Check sheet for the modelled part. Datum: model origin and axes. Units: mm. Face numbers are marked on the shaded views. A direction names the side the tool comes from. Give positions to 0.01 mm unless a question says otherwise; leave off trailing zeros. Loops run counter-clockwise (first coordinate to the right, second up) from the corner with the lowest first, then second, coordinate; pieces in that order, holes last. Notation, with made-up numbers: M -15,-25 L 13,-25 A20 ccw 13,-16 Z; hole C 31,18 d8. An arc over 180 degrees is marked long. Use one line per item in the form item = value.
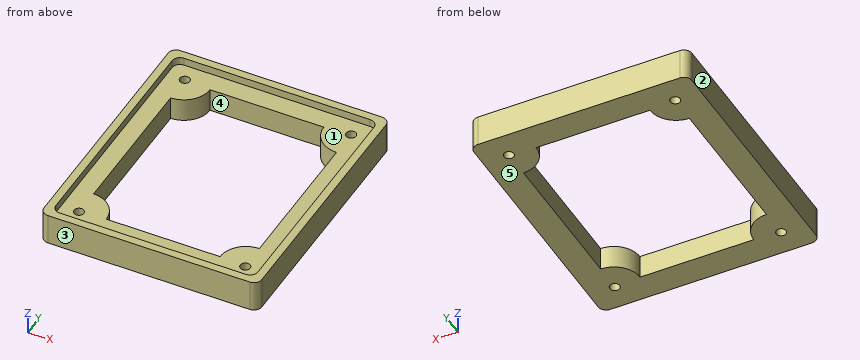
from build123d import *

# Parameters (mm, degrees)
F1_DEPTH = 6
F2_DEPTH = 8
F4_D     = 2.5
F4_DEPTH = 150
F4_TIP   = 0.7510757738
F5_R     = 2


with BuildPart() as f1:
    # F0 (on Top) → F1 (new body)
    with BuildSketch(Plane.XY):
        with BuildLine():
            Line((-20.9328360941, 18.9328360941), (-20.9328360941, 25.5))
            Line((-20.9328360941, 25.5), (-14.3656721882, 25.5))
            ThreePointArc((-14.3656721882, 25.5), (-14.9709415927, 28.2538074954), (-16.6751792541, 30.5))
            Line((-16.6751792541, 30.5), (-25.1904929341, 30.5))
            ThreePointArc((-25.1904929341, 30.5), (-25.3474833162, 30.3619473127), (-25.5, 30.2189676438))
            Line((-25.5, 30.2189676438), (-25.5, 20.7810323562))
            ThreePointArc((-25.5, 20.7810323562), (-23.3963100419, 19.4123947339), (-20.9328360941, 18.9328360941))
        make_face()
        with BuildLine():
            Line((-14.3656721882, 25.5), (-20.9328360941, 25.5))
            Line((-20.9328360941, 25.5), (-20.9328360941, 18.9328360941))
            ThreePointArc((-20.9328360941, 18.9328360941), (-16.289149963, 20.856313869), (-14.3656721882, 25.5))
        make_face()
        with BuildLine():
            ThreePointArc((-16.6751792541, 30.5), (-14.9709415927, 28.2538074954), (-14.3656721882, 25.5))
            Line((-14.3656721882, 25.5), (14.3656721882, 25.5))
            ThreePointArc((14.3656721882, 25.5), (14.9709415927, 28.2538074954), (16.6751792541, 30.5))
            Line((16.6751792541, 30.5), (-16.6751792541, 30.5))
        make_face()
        with BuildLine():
            ThreePointArc((16.6751792541, 30.5), (14.9709415927, 28.2538074954), (14.3656721882, 25.5))
            Line((14.3656721882, 25.5), (20.9328360941, 25.5))
            Line((20.9328360941, 25.5), (20.9328360941, 18.9328360941))
            ThreePointArc((20.9328360941, 18.9328360941), (23.3963100419, 19.4123947339), (25.5, 20.7810323562))
            Line((25.5, 20.7810323562), (25.5, 30.2189676438))
            ThreePointArc((25.5, 30.2189676438), (25.3474833162, 30.3619473127), (25.1904929341, 30.5))
            Line((25.1904929341, 30.5), (16.6751792541, 30.5))
        make_face()
        with BuildLine():
            Line((20.9328360941, 25.5), (14.3656721882, 25.5))
            ThreePointArc((14.3656721882, 25.5), (16.289149963, 20.856313869), (20.9328360941, 18.9328360941))
            Line((20.9328360941, 18.9328360941), (20.9328360941, 25.5))
        make_face()
        with BuildLine():
            ThreePointArc((25.5, 20.7810323562), (23.3963100419, 19.4123947339), (20.9328360941, 18.9328360941))
            Line((20.9328360941, 18.9328360941), (20.9328360941, -18.9328360941))
            ThreePointArc((20.9328360941, -18.9328360941), (23.3963100419, -19.4123947339), (25.5, -20.7810323562))
            Line((25.5, -20.7810323562), (25.5, 20.7810323562))
        make_face()
        with BuildLine():
            ThreePointArc((25.5, -20.7810323562), (23.3963100419, -19.4123947339), (20.9328360941, -18.9328360941))
            Line((20.9328360941, -18.9328360941), (20.9328360941, -25.5))
            Line((20.9328360941, -25.5), (14.3656721882, -25.5))
            ThreePointArc((14.3656721882, -25.5), (14.9709415927, -28.2538074954), (16.6751792541, -30.5))
            Line((16.6751792541, -30.5), (25.1904929341, -30.5))
            ThreePointArc((25.1904929341, -30.5), (25.3474833162, -30.3619473127), (25.5, -30.2189676438))
            Line((25.5, -30.2189676438), (25.5, -20.7810323562))
        make_face()
        with BuildLine():
            Line((20.9328360941, -25.5), (20.9328360941, -18.9328360941))
            ThreePointArc((20.9328360941, -18.9328360941), (16.289149963, -20.856313869), (14.3656721882, -25.5))
            Line((14.3656721882, -25.5), (20.9328360941, -25.5))
        make_face()
        with BuildLine():
            Line((-20.9328360941, -25.5), (-20.9328360941, -18.9328360941))
            ThreePointArc((-20.9328360941, -18.9328360941), (-23.3963100419, -19.4123947339), (-25.5, -20.7810323562))
            Line((-25.5, -20.7810323562), (-25.5, -30.2189676438))
            ThreePointArc((-25.5, -30.2189676438), (-25.3474833162, -30.3619473127), (-25.1904929341, -30.5))
            Line((-25.1904929341, -30.5), (-16.6751792541, -30.5))
            ThreePointArc((-16.6751792541, -30.5), (-14.9709415927, -28.2538074954), (-14.3656721882, -25.5))
            Line((-14.3656721882, -25.5), (-20.9328360941, -25.5))
        make_face()
        with BuildLine():
            ThreePointArc((-14.3656721882, -25.5), (-16.289149963, -20.856313869), (-20.9328360941, -18.9328360941))
            Line((-20.9328360941, -18.9328360941), (-20.9328360941, -25.5))
            Line((-20.9328360941, -25.5), (-14.3656721882, -25.5))
        make_face()
        with BuildLine():
            Line((-20.9328360941, -18.9328360941), (-20.9328360941, 18.9328360941))
            ThreePointArc((-20.9328360941, 18.9328360941), (-23.3963100419, 19.4123947339), (-25.5, 20.7810323562))
            Line((-25.5, 20.7810323562), (-25.5, -20.7810323562))
            ThreePointArc((-25.5, -20.7810323562), (-23.3963100419, -19.4123947339), (-20.9328360941, -18.9328360941))
        make_face()
        with BuildLine():
            Line((14.3656721882, -25.5), (-14.3656721882, -25.5))
            ThreePointArc((-14.3656721882, -25.5), (-14.9709415927, -28.2538074954), (-16.6751792541, -30.5))
            Line((-16.6751792541, -30.5), (16.6751792541, -30.5))
            ThreePointArc((16.6751792541, -30.5), (14.9709415927, -28.2538074954), (14.3656721882, -25.5))
        make_face()
        with BuildLine():
            Line((25.5, 30.5), (25.1904929341, 30.5))
            ThreePointArc((25.1904929341, 30.5), (25.3474833162, 30.3619473127), (25.5, 30.2189676438))
            Line((25.5, 30.2189676438), (25.5, 30.5))
        make_face()
        with BuildLine():
            ThreePointArc((-25.5, 30.2189676438), (-25.3474833162, 30.3619473127), (-25.1904929341, 30.5))
            Line((-25.1904929341, 30.5), (-25.5, 30.5))
            Line((-25.5, 30.5), (-25.5, 30.2189676438))
        make_face()
        with BuildLine():
            ThreePointArc((-25.1904929341, -30.5), (-25.3474833162, -30.3619473127), (-25.5, -30.2189676438))
            Line((-25.5, -30.2189676438), (-25.5, -30.5))
            Line((-25.5, -30.5), (-25.1904929341, -30.5))
        make_face()
        with BuildLine():
            Line((25.5, -30.5), (25.5, -30.2189676438))
            ThreePointArc((25.5, -30.2189676438), (25.3474833162, -30.3619473127), (25.1904929341, -30.5))
            Line((25.1904929341, -30.5), (25.5, -30.5))
        make_face()
    extrude(amount=F1_DEPTH)

    # F0 (on Top) → F2 (join)
    with BuildSketch(Plane.XY):
        with BuildLine():
            ThreePointArc((-25.1904929341, 30.5), (-20.9328360941, 32.0671639059), (-16.6751792541, 30.5))
            Line((-16.6751792541, 30.5), (16.6751792541, 30.5))
            ThreePointArc((16.6751792541, 30.5), (20.9328360941, 32.0671639059), (25.1904929341, 30.5))
            Line((25.1904929341, 30.5), (25.5, 30.5))
            Line((25.5, 30.5), (25.5, 30.2189676438))
            ThreePointArc((25.5, 30.2189676438), (26.9793621927, 28.062647831), (27.5, 25.5))
            Line((27.5, 25.5), (27.5, 32.5))
            Line((27.5, 32.5), (-27.5, 32.5))
            Line((-27.5, 32.5), (-27.5, 25.5))
            ThreePointArc((-27.5, 25.5), (-26.9793621927, 28.062647831), (-25.5, 30.2189676438))
            Line((-25.5, 30.2189676438), (-25.5, 30.5))
            Line((-25.5, 30.5), (-25.1904929341, 30.5))
        make_face()
        with BuildLine():
            Line((-25.1904929341, 30.5), (-16.6751792541, 30.5))
            ThreePointArc((-16.6751792541, 30.5), (-20.9328360941, 32.0671639059), (-25.1904929341, 30.5))
        make_face()
        with BuildLine():
            ThreePointArc((-27.5, 25.5), (-26.9793621927, 22.937352169), (-25.5, 20.7810323562))
            Line((-25.5, 20.7810323562), (-25.5, 30.2189676438))
            ThreePointArc((-25.5, 30.2189676438), (-26.9793621927, 28.062647831), (-27.5, 25.5))
        make_face()
        with BuildLine():
            Line((-25.5, -20.7810323562), (-25.5, 20.7810323562))
            ThreePointArc((-25.5, 20.7810323562), (-26.9793621927, 22.937352169), (-27.5, 25.5))
            Line((-27.5, 25.5), (-27.5, -25.5))
            ThreePointArc((-27.5, -25.5), (-26.9793621927, -22.937352169), (-25.5, -20.7810323562))
        make_face()
        with BuildLine():
            Line((-25.5, -30.2189676438), (-25.5, -20.7810323562))
            ThreePointArc((-25.5, -20.7810323562), (-26.9793621927, -22.937352169), (-27.5, -25.5))
            ThreePointArc((-27.5, -25.5), (-26.9793621927, -28.062647831), (-25.5, -30.2189676438))
        make_face()
        with BuildLine():
            Line((16.6751792541, -30.5), (-16.6751792541, -30.5))
            ThreePointArc((-16.6751792541, -30.5), (-20.9328360941, -32.0671639059), (-25.1904929341, -30.5))
            Line((-25.1904929341, -30.5), (-25.5, -30.5))
            Line((-25.5, -30.5), (-25.5, -30.2189676438))
            ThreePointArc((-25.5, -30.2189676438), (-26.9793621927, -28.062647831), (-27.5, -25.5))
            Line((-27.5, -25.5), (-27.5, -32.5))
            Line((-27.5, -32.5), (27.5, -32.5))
            Line((27.5, -32.5), (27.5, -25.5))
            ThreePointArc((27.5, -25.5), (26.9793621927, -28.062647831), (25.5, -30.2189676438))
            Line((25.5, -30.2189676438), (25.5, -30.5))
            Line((25.5, -30.5), (25.1904929341, -30.5))
            ThreePointArc((25.1904929341, -30.5), (20.9328360941, -32.0671639059), (16.6751792541, -30.5))
        make_face()
        with BuildLine():
            ThreePointArc((-25.1904929341, -30.5), (-20.9328360941, -32.0671639059), (-16.6751792541, -30.5))
            Line((-16.6751792541, -30.5), (-25.1904929341, -30.5))
        make_face()
        with BuildLine():
            Line((25.1904929341, -30.5), (16.6751792541, -30.5))
            ThreePointArc((16.6751792541, -30.5), (20.9328360941, -32.0671639059), (25.1904929341, -30.5))
        make_face()
        with BuildLine():
            ThreePointArc((27.5, -25.5), (26.9793621927, -22.937352169), (25.5, -20.7810323562))
            Line((25.5, -20.7810323562), (25.5, -30.2189676438))
            ThreePointArc((25.5, -30.2189676438), (26.9793621927, -28.062647831), (27.5, -25.5))
        make_face()
        with BuildLine():
            ThreePointArc((25.1904929341, 30.5), (20.9328360941, 32.0671639059), (16.6751792541, 30.5))
            Line((16.6751792541, 30.5), (25.1904929341, 30.5))
        make_face()
        with BuildLine():
            Line((25.5, 30.2189676438), (25.5, 20.7810323562))
            ThreePointArc((25.5, 20.7810323562), (26.9793621927, 22.937352169), (27.5, 25.5))
            ThreePointArc((27.5, 25.5), (26.9793621927, 28.062647831), (25.5, 30.2189676438))
        make_face()
        with BuildLine():
            ThreePointArc((27.5, 25.5), (26.9793621927, 22.937352169), (25.5, 20.7810323562))
            Line((25.5, 20.7810323562), (25.5, -20.7810323562))
            ThreePointArc((25.5, -20.7810323562), (26.9793621927, -22.937352169), (27.5, -25.5))
            Line((27.5, -25.5), (27.5, 25.5))
        make_face()
    extrude(amount=F2_DEPTH)

    # F4
    with Locations(Plane.XY.offset(6)):
        with Locations((-21, 26), (21, 26), (21, -26), (-21, -26)):
            Hole(F4_D / 2, depth=F4_DEPTH)
            with Locations((0, 0, -(F4_DEPTH + F4_TIP / 2))):  # 118° drill point
                Cone(0, F4_D / 2, F4_TIP, mode=Mode.SUBTRACT)

    # F5
    f5_edges = [f1.edges().sort_by_distance(p)[0] for p in [
        (25.5, 30.5, 7),
        (25.5, -30.5, 7),
        (-25.5, -30.5, 7),
        (-25.5, 30.5, 7),
        (27.5, 32.5, 4),
        (27.5, -32.5, 4),
        (-27.5, -32.5, 4),
        (-27.5, 32.5, 4),
    ]]
    fillet(f5_edges, radius=F5_R)


solid = f1.part
1) Release check for a two-part mould opening along Y. For the marked faces 1, 2 and 3 record: pulls with the +Y half, pulls with the -Y half, needs draft (parallel to the pull), parting line crosses it, or undercut.
Evaluation:
face_1 = undercut
face_2 = needs draft
face_3 = pulls with the -Y half
2) Scan lines: line 1 (Y direction, x = -21, z = 1.3); line 2 (X direction, y = -25.5, z = 6.75); line 3 (Y direction, x = 3, z = 3.5). Record each from-to range of solid material in increasing order.
Evaluation:
line_1 = -32.5 to -27.25, -24.75 to 24.75, 27.25 to 32.5
line_2 = -27.5 to -25.5, 25.5 to 27.5
line_3 = -32.5 to -25.5, 25.5 to 32.5
3) Set-up check for the marked faces 4 and 5: record each of +Z, -Z, +X, -X, +Y, -Y from which the full face is reachable in a straight line by a thin tool's end or side.
Evaluation:
face_4 = +Z, -Z
face_5 = -Z, +X, -X, +Y, -Y
4) Section check A-A (y = -3.5). Record the cut outline in (x, z).
Evaluation:
outline = M -27.5,0 L -20.93,0 L -20.93,6 L -25.5,6 L -25.5,8 L -27.5,8 Z; M 20.93,0 L 27.5,0 L 27.5,8 L 25.5,8 L 25.5,6 L 20.93,6 Z
5) Depth check by flat-ended pin: pin 1 Ø2 at (x, y) = (21, 26) entering from -Z; pin 2 Ø3 at (x, y) = (21, -26) entering from +Z. Enter the tip coordinate at first touch or a pass-through.
Evaluation:
pin_1 = through
pin_2 = 6
6) Section check C-C (z = 1.5). Record the cut outline in (x, y), then the cut area to 3 significant figures.
Evaluation:
outline = M -27.5,-30.5 A2 ccw -25.5,-32.5 L 25.5,-32.5 A2 ccw 27.5,-30.5 L 27.5,30.5 A2 ccw 25.5,32.5 L -25.5,32.5 A2 ccw -27.5,30.5 Z; hole C -21,-26 d2.5; hole C -21,26 d2.5; hole M -20.93,-18.93 A6.57 cw -14.37,-25.5 L 14.37,-25.5 A6.57 cw 20.93,-18.93 L 20.93,18.93 A6.57 cw 14.37,25.5 L -14.37,25.5 A6.57 cw -20.93,18.93 Z; hole C 21,-26 d2.5; hole C 21,26 d2.5
area = 1,550 mm^2
7) Section check B-B (x = 6). Record the cut outline in (y, z).
Evaluation:
outline = M -32.5,0 L -25.5,0 L -25.5,6 L -30.5,6 L -30.5,8 L -32.5,8 Z; M 25.5,0 L 32.5,0 L 32.5,8 L 30.5,8 L 30.5,6 L 25.5,6 Z
